Build history of the part. All positions in model axes, mm. Round coordinates to 2 decimals unless told otherwise and drop trailing zeros. Write each loop counter-clockwise with the first axis right and the second up, starting at its lowest first coordinate (ties: lowest second). Pieces come first, ordered by that corner, then holes. Notation, with made-up numbers: M 89.5,29.5 L 127.5,29.5 A15 ccw 127.5,48.5 Z; hole C 4.5,-2.5 d8. An arc over 180 degrees is marked long. Use a Markdown table: item, result.
Autodesk Inventor part; units mm, degrees
ref_plane "YZ Plane" through (0, 0, 0) normal (1, 0, 0) x (0, 1, 0)
ref_plane "XZ Plane" through (0, 0, 0) normal (0, 1, 0) x (-1, 0, 0)
ref_plane "XY Plane" through (0, 0, 0) normal (0, 0, 1) x (1, 0, 0)
sketch "Sketch1" plane through (0, 0, 0) normal (0, 0, 1) x (1, 0, 0)
  circle A0 centre (0, 0) radius 20.32
  circle A1 centre (31.75, 0) radius 38.1
  line L0 (31.75, 0) -> (4.8092, 26.9408)
  line L1 (31.75, 0) -> (4.8092, -26.9408)
  dimension "d0" = 40.64
  dimension "d1" = 90
  dimension "d3" = 0
  dimension "d5" = 31.75
  dimension "d6" = 76.2
extrude "Extrusion1" add sketch "Sketch1" along normal blind 3.175 contours A1 L1 L0
sketch "Sketch2" plane through (0, 0, 3.175) normal (0, 0, 1) x (1, 0, 0)
  line L0 (31.75, 0) -> (4.8092, -26.9408)
  circle A0 centre (31.75, 0) radius 1.5875
  circle A1 centre (31.75, 0) radius 3.175
  point P0 (0, 0)
  dimension "d10" = 3.175
  dimension "d11" = 6.35
extrude "Extrusion2" add sketch "Sketch2" against normal blind 3.175
sketch "Sketch3" plane through (0, 0, 3.175) normal (0, 0, 1) x (1, 0, 0)
  line L0 (31.75, 0) -> (30.6275, -1.1225)
  circle A0 centre (31.75, 0) radius 1.5875
  point P0 (0, 0)
extrude "Extrusion3" cut sketch "Sketch3" against normal blind 3.175
properties part number "Release1"
Q1. Cut at D-D on y = -24. Give the cut face in (x, z) (3 decimals), and give its area (3 significant figures).
Response values:
| item | result |
|---|---|
| outline | M 7.75,0 L 61.341,0 L 61.341,3.175 L 7.75,3.175 Z |
| area | 170 mm2 |
Q2. Cut at B-B on x = 31.75. Give the cut face in (y, z) (1 decimal).
Response values:
| item | result |
|---|---|
| outline | M -38.1,0 L -1.6,0 L -1.6,3.2 L -38.1,3.2 Z; M 1.6,0 L 38.1,0 L 38.1,3.2 L 1.6,3.2 Z |
Q3. Two-plate mould, pull along Y, no slides. Class faces 1 (the flat face through (17.33, 14.42, 1.57)), 2 (the flat face through (17.33, -14.42, 1.57)), 3 (the cylindrical face through (69.83, 1.26, 1.57)), 4 (the flat face through (37, 1, 0)): +Y half, -Y half, draft (parallel to the pull), parting line (faces both ways), or undercut.
Response values:
| item | result |
|---|---|
| face 1 | undercut |
| face 2 | undercut |
| face 3 | parting line |
| face 4 | draft |
Q4. Drop a flat-ended pin along its axis: P1, Ø1, axis at y = 1, z = 1, coming from the +X side. Give the stop position or say it passes through.
Response values:
| item | result |
|---|---|
| P1 | stops at x = 69.85 |
Q5. Drill centre lines: L1, parallel to Y at x = 31.75, z = 0.7; L2, parallel to Y at x = 26, z = 1.3; L3, parallel to X at y = 24, z = 2.8. Where is each one in solid material? Low to high.
Response values:
| item | result |
|---|---|
| L1 | y = -38.1 to -1.59, 1.59 to 38.1 |
| L2 | y = -37.66 to -5.75, 5.75 to 37.66 |
| L3 | x = 7.75 to 61.34 |
